CAD build for the part. Positions are in the model's coordinates, mm. Give positions to 0.01 mm unless a question says otherwise; leave off trailing zeros. Loops run counter-clockwise (first coordinate to the right, second up) from the corner with the lowest first, then second, coordinate; pieces in that order, holes last.
Item 1: Saw through at B-B on x = 115. Give the cut face in (y, z), plus the area to 3 significant figures.
Item 2: Saw through at A-A on y = 12. Give the cut face in (x, z).
Item 3: Drop flat-ended pins along their axis: P1, Ø0.5, axis at x = -37.5, y = 21, coming from the -Z side; P2, Ø1.5, axis at x = -186, z = 6.5, coming from the -Y side; P3, Ø5, axis at x = 202.5, z = 11, coming from the -Y side; P4, Ø2, axis at x = -5.5, z = 12.5, coming from the -Y side. Give the stop position or say it passes through.
Item 4: Saw through at C-C on z = 7.62. Give the cut face in (x, y), plus the area to 3 significant figures.
Item 5: Probe probe 1 along Z at (x, y) = (-143, 14); probe 2 along Z at (x, y) = (115.5, 21.25); probe 3 along Z at (x, y) = (174, 2). List the from-to ranges inside material, lowest first.
from build123d import *

# Parameters (mm, degrees)
BOSS_EXTRUDE1_DEPTH         = 278.60625
CUT_FRONT_LEFT_BOTTOM_DEPTH = 16.24
CUT_TOP_RIGHT_FRONT_DEPTH   = 22.844


with BuildPart() as part:
    # Sketch1 → Boss-Extrude1 (new body, symmetric)
    with BuildSketch(Plane(origin=(0, 0, 0), x_dir=(0, 0, -1), z_dir=(1, 0, 0))):
        with BuildLine():
            Line((0, 0), (0, 21.844))
            Line((0, 21.844), (-5.08, 21.844))
            Line((-5.08, 21.844), (-5.08, 20.066))
            ThreePointArc((-5.08, 20.066), (-7.62, 17.526), (-10.16, 20.066))
            Line((-10.16, 20.066), (-10.16, 21.844))
            Line((-10.16, 21.844), (-15.24, 21.844))
            Line((-15.24, 21.844), (-15.24, 3.048))
            Line((-15.24, 3.048), (-13.97, 3.048))
            Line((-13.97, 3.048), (-13.97, 20.574))
            Line((-13.97, 20.574), (-11.43, 20.574))
            Line((-11.43, 20.574), (-11.43, 20.066))
            ThreePointArc((-11.43, 20.066), (-7.62, 16.256), (-3.81, 20.066))
            Line((-3.81, 20.066), (-3.81, 20.574))
            Line((-3.81, 20.574), (-1.27, 20.574))
            Line((-1.27, 20.574), (-1.27, 0))
            Line((-1.27, 0), (0, 0))
        make_face()
    extrude(amount=BOSS_EXTRUDE1_DEPTH, both=True)

    # Sketch7 → Cut-Front-Left-Bottom (cut, through all)
    with BuildSketch(Plane.XY.offset(15.24)):
        Polygon((-278.60625, 21.844), (-256.76225, 0), (-278.60625, 0), align=None)
    extrude(amount=-CUT_FRONT_LEFT_BOTTOM_DEPTH, mode=Mode.SUBTRACT)

    # Sketch2 → Cut-Top-Right-Front (cut, through all)
    with BuildSketch(Plane(origin=(0, 21.844, 0), x_dir=(1, 0, 0), z_dir=(0, 1, 0))):
        Polygon((278.60625, 0), (263.36625, -15.24), (278.60625, -15.24), align=None)
    extrude(amount=-CUT_TOP_RIGHT_FRONT_DEPTH, mode=Mode.SUBTRACT)


solid = part.part
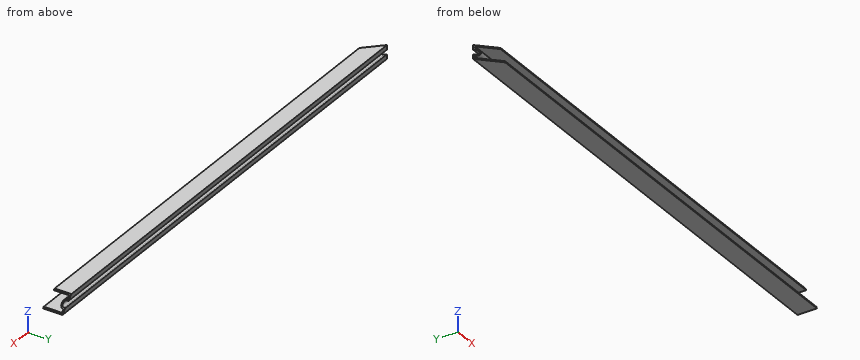
Results below:
1. outline: (0, 0) - (21.84, 0) - (21.84, 5.08) - (20.07, 5.08) arc R2.54 cw to (20.07, 10.16) - (21.84, 10.16) - (21.84, 15.24) - (3.05, 15.24) - (3.05, 13.97) - (20.57, 13.97) - (20.57, 11.43) - (20.07, 11.43) arc R3.81 ccw to (20.07, 3.81) - (20.57, 3.81) - (20.57, 1.27) - (0, 1.27) - close
1. area: 75.2 mm2
2. outline: (-268.76, 0) - (278.61, 0) - (277.34, 1.27) - (-268.76, 1.27) - close; (-268.76, 13.97) - (264.64, 13.97) - (263.37, 15.24) - (-268.76, 15.24) - close
3. P1: stops at z = 0
3. P2: stops at y = 16.27
3. P3: stops at y = 16.36
3. P4: stops at y = 20.57
4. outline: (-274.29, 17.53) - (-273.02, 16.26) - (270.99, 16.26) - (270.99, 17.53) - close
4. area: 692 mm2
5. probe 1: z = 0 to 1.27, 13.97 to 15.24
5. probe 2: z = 0 to 5.08, 10.16 to 15.24
5. probe 3: z = 0 to 1.27
